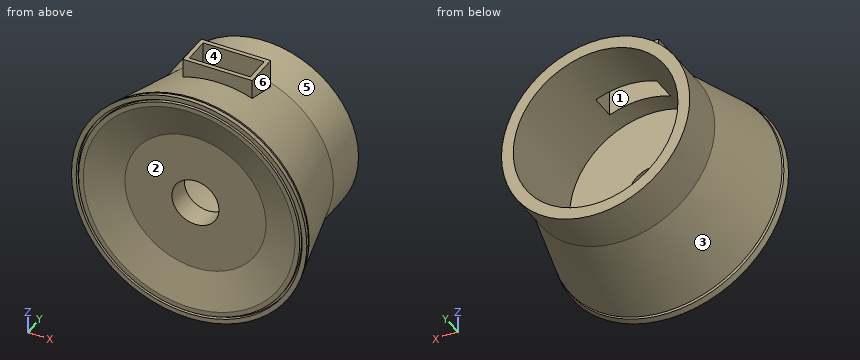
```python
from build123d import *

# Parameters (mm, degrees)
SKETCH1_R           = 25
BOSS_EXTRUDE1_DEPTH = 30
SKETCH3_W           = 5
SKETCH3_H           = 17.5
SKETCH3_W_2         = 0.5
SKETCH3_H_2         = 0.75
SKETCH6_W           = 14.74
SKETCH6_H           = 7.36
SKETCH6_W_2         = 12.96
SKETCH6_H_2         = 5.56
BOSS_EXTRUDE2_DEPTH = 25
SKETCH4_R           = 17.5
CUT_EXTRUDE1_DEPTH  = 22.5
SKETCH6_5_W         = 12.96
SKETCH6_5_H         = 5.56
CUT_EXTRUDE7_DEPTH  = 46.5


with BuildPart() as part:
    # Sketch1 → Boss-Extrude1 (new body)
    with BuildSketch(Plane(origin=(0, 0, 0), x_dir=(1, 0, 0), z_dir=(0, 1, 0))):
        Circle(SKETCH1_R)
    extrude(amount=BOSS_EXTRUDE1_DEPTH)

    # Sketch3 → Cut-Revolve1 (revolve, cut)
    with BuildSketch(Plane.XY):
        Polygon((-24.5625, 1.75), (-20, 20), (-20, 30), (-25, 30), (-25, 20), (-25, 0), (-24.6875, 1.25), (-23.75, 1.25), (-23.75, 1.75), align=None)
        Polygon((0, 0), (0, 2.5), (-5, 2.5), (-15, 2.5), (-22.5, 0), (-15, 0), align=None)
        with Locations((-2.5, 11.25)):
            Rectangle(SKETCH3_W, SKETCH3_H)
        with Locations((-23.75, 0.375)):
            Rectangle(SKETCH3_W_2, SKETCH3_H_2)
    revolve(axis=Axis((0, 31.461521879, 0), (0, -1, 0)), mode=Mode.SUBTRACT)

    # Sketch6 → Boss-Extrude2 (add)
    with BuildSketch(Plane.XY):
        with Locations((0, 15)):
            Rectangle(SKETCH6_W, SKETCH6_H)
        with Locations((0, 15)):
            Rectangle(SKETCH6_W_2, SKETCH6_H_2, mode=Mode.SUBTRACT)
    extrude(amount=BOSS_EXTRUDE2_DEPTH)

    # Sketch4 → Cut-Extrude1 (cut)
    with BuildSketch(Plane(origin=(0, 30, 0), x_dir=(1, 0, 0), z_dir=(0, 1, 0))):
        Circle(SKETCH4_R)
    extrude(amount=-CUT_EXTRUDE1_DEPTH, mode=Mode.SUBTRACT)

    # Sketch6_5 → Cut-Extrude7 (cut)
    with BuildSketch(Plane.XY):
        with Locations((0, 15)):
            Rectangle(SKETCH6_5_W, SKETCH6_5_H)
    extrude(amount=CUT_EXTRUDE7_DEPTH, mode=Mode.SUBTRACT)


solid = part.part
```
For this review, take the finished solid that the model builds, in its own axes (mm). Face numbers are marked on the shaded views. A direction names the side the tool comes from. Coordinates: 2 decimals unless noted, no trailing zeros. Write each loop counter-clockwise with the first axis right and the second up, starting at its lowest first coordinate (ties: lowest second). Pieces come first, ordered by that corner, then holes.
(1) For pin 1 Ø3 at (y, z) = (13.5, 21.5) entering from +X; pin 2 Ø1.5 at (x, z) = (-6, -6.5) entering from +Y; pin 3 Ø4 at (y, z) = (16.5, 0) entering from +X (3 decimals), all flat-tipped, find the tip position at first contact; note any pin that passes through.
(2) Add section B-B on y = 15.5. Give the boundary of the cut face in (x, z) (3 decimals).
(3) Add section C-C on x = 0. Count the separate pieces of the cut face and the enclosed holes in it, then the cut area to 3 significant figures.
(4) The part is to be moulded in two halves that separate along Z. For the marked faces 1, 2 and 3, say which applies: +Z half, -Z half, draft (parallel to the pull), parting line (faces both ways), or undercut.
(5) Wall thickness on probe 1 along Z at (x, y) = (0, 20.75); probe 2 along Y at (x, z) = (-1.5, -13); probe 3 along X at (y, z) = (4.2, 0): over which ranges is each line inside the solid? List them lowest first.
(6) Tool access review of the marked faces 4, 5 and 6: name each direction out of +Z, -Z, +X, -X, +Y, -Y from which nothing blocks a thin tool from reaching the whole face with its end or side.
Answer sheet:
1. pin 1: stops at x = 8.35
1. pin 2: stops at y = 7.5
1. pin 3: stops at x = 21.375
2. outline: (-7.37, 19.798) arc R21.125 ccw (long way) to (7.37, 19.798) - (7.37, 25) - (6.48, 25) - (6.48, 16.256) arc R17.5 cw (long way) to (-6.48, 16.256) - (-6.48, 25) - (-7.37, 25) - close
3. separate pieces: 3
3. enclosed holes: 0
3. area: 353 mm2
4. face 1: draft
4. face 2: undercut
4. face 3: parting line
5. probe 1: z = -20 to -17.5, 17.5 to 20
5. probe 2: y = 2.5 to 7.5
5. probe 3: x = -23.95 to -5, 5 to 23.95
6. face 4: +Z
6. face 5: +Y
6. face 6: +Z, +X, +Y
